Check sheet for the modelled part. Datum: model origin and axes. Units: mm. Face numbers are marked on the shaded views. A direction names the side the tool comes from. Round coordinates to 2 decimals unless told otherwise and drop trailing zeros. Write each loop counter-clockwise with the first axis right and the second up, starting at its lowest first coordinate (ties: lowest second). Pieces come first, ordered by that corner, then holes.
Item 1: Go/stop test with flat-tipped pins: pin 1 Ø8 at (y, z) = (-19, 12) entering from +X; pin 2 Ø2 at (x, z) = (15, 10) entering from +Y; pin 3 Ø12 at (y, z) = (32, 18) entering from +X. Record where each tip stops, or that it passes through.
Item 2: Release check for a two-part mould opening along X. For the marked faces 3, 4, 5 and 6 record: +X half, -X half, draft (parallel to the pull), parting line (faces both ways), or undercut.
Item 3: Material ranges on line 1 (Z direction, x = -11, y = -26); line 2 (X direction, y = -38.5, z = 20.25); line 3 (Y direction, x = 8.5, z = 4), recorded low to high.
Item 4: Cross-section at A-A on x = -10. Enter the section's corners in (y, z), plus the area to 3 significant figures.
Item 5: Cross-section at D-D on z = 18.75. Enter the section's corners in (x, y), plus the area to 3 significant figures.
Item 6: Tool access check on the marked faces 1 and 2. Record the directions out of +Z, -Z, +X, -X, +Y, -Y that give a thin tool (end or side, any length) a straight path to the whole face; none if there is none.
Item 7: Cross-section at B-B on z = 7. Enter the section's corners in (x, y), plus the area to 3 significant figures.
Item 8: Cross-section at C-C on y = -39. Enter the section's corners in (x, z), plus the area to 3 significant figures.
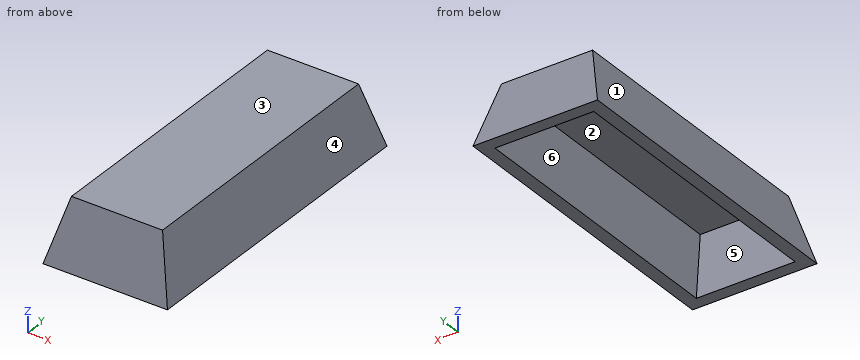
from build123d import *

# Parameters (mm, degrees)
F0_W     = 50.8
F0_H     = 127
F1_DEPTH = 25.4
F1_TAPER = 15
F2_T     = -5.08


with BuildPart() as f1:
    # F0 (on Top) → F1 (new body)
    with BuildSketch(Plane.XY):
        Rectangle(F0_W, F0_H)
    extrude(amount=F1_DEPTH, taper=F1_TAPER)

    # F2
    f2_openings = [f1.faces().sort_by_distance(p)[0] for p in [
        (0, 0, 0),
    ]]
    offset(amount=F2_T, openings=f2_openings)


solid = f1.part
Response values:
1. pin 1: stops at x = 23.26
1. pin 2: stops at y = 61.09
1. pin 3: stops at x = 22.18
2. face 3: draft
2. face 4: +X half
2. face 5: undercut
2. face 6: undercut
3. line 1: z = 20.32 to 25.4
3. line 2: x = -19.97 to -14.71, 14.71 to 19.97
3. line 3: y = -62.43 to -57.17, 57.17 to 62.43
4. outline: (-63.5, 0) - (-58.24, 0) - (-52.8, 20.32) - (52.8, 20.32) - (58.24, 0) - (63.5, 0) - (56.69, 25.4) - (-56.69, 25.4) - close
4. area: 797 mm2
5. outline: (-20.38, -58.48) - (20.38, -58.48) - (20.38, 58.48) - (-20.38, 58.48) - close; hole (-15.12, -53.22) - (15.12, -53.22) - (15.12, 53.22) - (-15.12, 53.22) - close
5. area: 1,550 mm2
6. face 1: +Z, -X, +Y, -Y
6. face 2: -Z
7. outline: (-23.52, -61.62) - (23.52, -61.62) - (23.52, 61.62) - (-23.52, 61.62) - close; hole (-18.27, -56.37) - (18.27, -56.37) - (18.27, 56.37) - (-18.27, 56.37) - close
7. area: 1,680 mm2
8. outline: (-25.4, 0) - (-20.14, 0) - (-14.7, 20.32) - (14.7, 20.32) - (20.14, 0) - (25.4, 0) - (18.59, 25.4) - (-18.59, 25.4) - close
8. area: 410 mm2
